Build history of the part. All positions in model axes, mm. Face numbers are marked on the shaded views. A direction names the side the tool comes from. Round coordinates to 2 decimals unless told otherwise and drop trailing zeros. Order: outer loops, then holes, each group sorted by start corner. A loop starts at its lowest first (then second) coordinate and runs counter-clockwise, first axis right, second up. Notation, with made-up numbers: (13.5, -16.5) -> (46.5, -16.5) arc R20 ccw to (46.5, 11.5) -> close; hole circle Ø1 at (45.25, 23.25). An arc over 180 degrees is marked (long way). Write item = value, one per line.
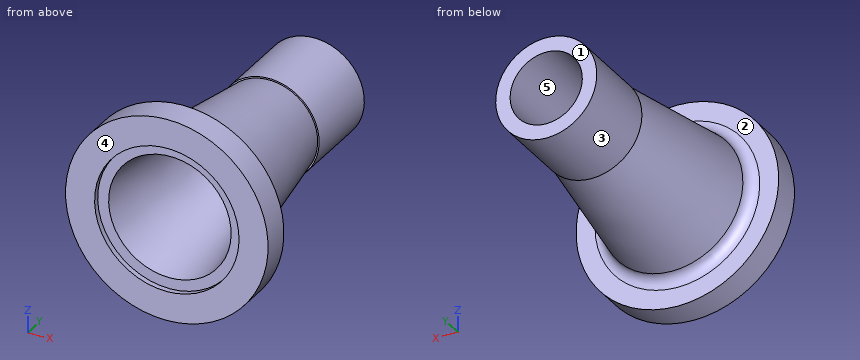
from build123d import *

# Parameters (mm, degrees)
FILLET1_R = 8


with BuildPart() as part:
    # Sketch3 → Revolve1 (revolve)
    with BuildSketch(Plane.XY, mode=Mode.PRIVATE) as revolve1_sk:
        Polygon((25, 185.89945678), (35, 185.89945678), (35, 128.787624663), (33.963762469, 128.787624663), (50.124510314, 20), (70.124510314, 20), (70.124510314, 0), (50, 0), (50, 3.89945678), (42.40655913, 3.89945678), (25, 121.073379639), align=None)
    revolve(revolve1_sk.sketch.rotate(Axis((0, 0, 0), (0, 1, 0)), 90), axis=Axis((0, 0, 0), (0, 1, 0)))

    # Fillet1
    fillet1_edges = [part.edges().sort_by_distance(p)[0] for p in [
        (0, 20, 50.124510314),
    ]]
    fillet(fillet1_edges, radius=FILLET1_R)


solid = part.part
Q1. Cut at B-B, the plane z = 0. List the corners of the cut face in (x, y), and give its area (3 significant figures).
Check values:
outline = (-70.12, 0) -> (-50, 0) -> (-50, 3.9) -> (-42.41, 3.9) -> (-25, 121.07) -> (-25, 185.9) -> (-35, 185.9) -> (-35, 128.79) -> (-33.96, 128.79) -> (-49.11, 26.82) arc R8 cw to (-57.02, 20) -> (-70.12, 20) -> close; (25, 121.07) -> (42.41, 3.9) -> (50, 3.9) -> (50, 0) -> (70.12, 0) -> (70.12, 20) -> (57.02, 20) arc R8 cw to (49.11, 26.82) -> (33.96, 128.79) -> (35, 128.79) -> (35, 185.9) -> (25, 185.9) -> close
area = 4,440 mm²
Q2. Probe probe 1 along X at (y, z) = (2.6, 0); probe 2 along Y at (x, z) = (21, 62.5); probe 3 along X at (y, z) = (25.5, 9.5). List the from-to ranges inside material, lowest first.
Check values:
probe_1 = -70.12 to -50, 50 to 70.12
probe_2 = 0 to 20
probe_3 = -48.5 to -38.03, 38.03 to 48.5
Q3. Cut at A-A, the plane x = 0. List the corners of the cut face in (y, z).
Check values:
outline = (0, -70.12) -> (20, -70.12) -> (20, -57.02) arc R8 cw to (26.82, -49.11) -> (128.79, -33.96) -> (128.79, -35) -> (185.9, -35) -> (185.9, -25) -> (121.07, -25) -> (3.9, -42.41) -> (3.9, -50) -> (0, -50) -> close; (0, 50) -> (3.9, 50) -> (3.9, 42.41) -> (121.07, 25) -> (185.9, 25) -> (185.9, 35) -> (128.79, 35) -> (128.79, 33.96) -> (26.82, 49.11) arc R8 cw to (20, 57.02) -> (20, 70.12) -> (0, 70.12) -> close
Q4. Which spindle directions (+Z, -Z, +X, -X, +Y, -Y) get a long thin tool onto all of the face, cutting with end or side? Do the marked faces 1 and 2. Say none if no direction does.
Check values:
face_1 = +Z, -Z, +X, -X, +Y
face_2 = +Y
Q5. Cut at C-C, the plane y = 133.5. List the corners of the cut face in (x, z), and give its area (3 significant figures).
Check values:
outline = circle Ø70 at (0, 0); hole circle Ø50 at (0, 0)
area = 1,880 mm²
Q6. Mould opens along Z. For the marked faces 3, 4 and 5 say: released by +Z, released by -Z, zero draft, split by the parting line, or undercut.
Check values:
face_3 = split by the parting line
face_4 = zero draft
face_5 = undercut
Q7. Flat gauge pins, fed straight in: pin 1 (12 mm diameter, centred on x = -39.5, z = -6.5, fed in from -Y); pin 2 (12 mm diameter, centred on x = 22.5, y = 144.5, fed in from -Z); pin 3 (10 mm diameter, centred on x = -31, y = 28.5, fed in from +Z); pin 4 (5 mm diameter, centred on x = 45.5, z = 51, fed in from -Y). Where does each tip first touch, or does it go through?
Check values:
pin_1 = 3.9
pin_2 = -30.87
pin_3 = 41.49
pin_4 = 0
Q8. Cut at D-D, the plane y = 61. List the corners of the cut face in (x, z), and give its area (3 significant figures).
Check values:
outline = circle Ø88.07 at (0, 0); hole circle Ø67.85 at (0, 0)
area = 2,480 mm²
